The figure shows three views and two pictorial views of one solid part (mm, origin at its lowest corner). Answer the questions. A direction names the side the tool comes from. Give positions to 0.01 mm unless a question says otherwise; leave off trailing zeros. Loops run counter-clockwise (first coordinate to the right, second up) from the corner with the lowest first, then second, coordinate; pieces in that order, holes last. Notation, with made-up numbers: (-6.75, 79.5) - (2.25, 79.5) arc R17 ccw to (2.25, 100.5) - close; hole circle Ø10 at (7, 68). An arc over 180 degrees is marked (long way). One line per question, with ' | ' between items.
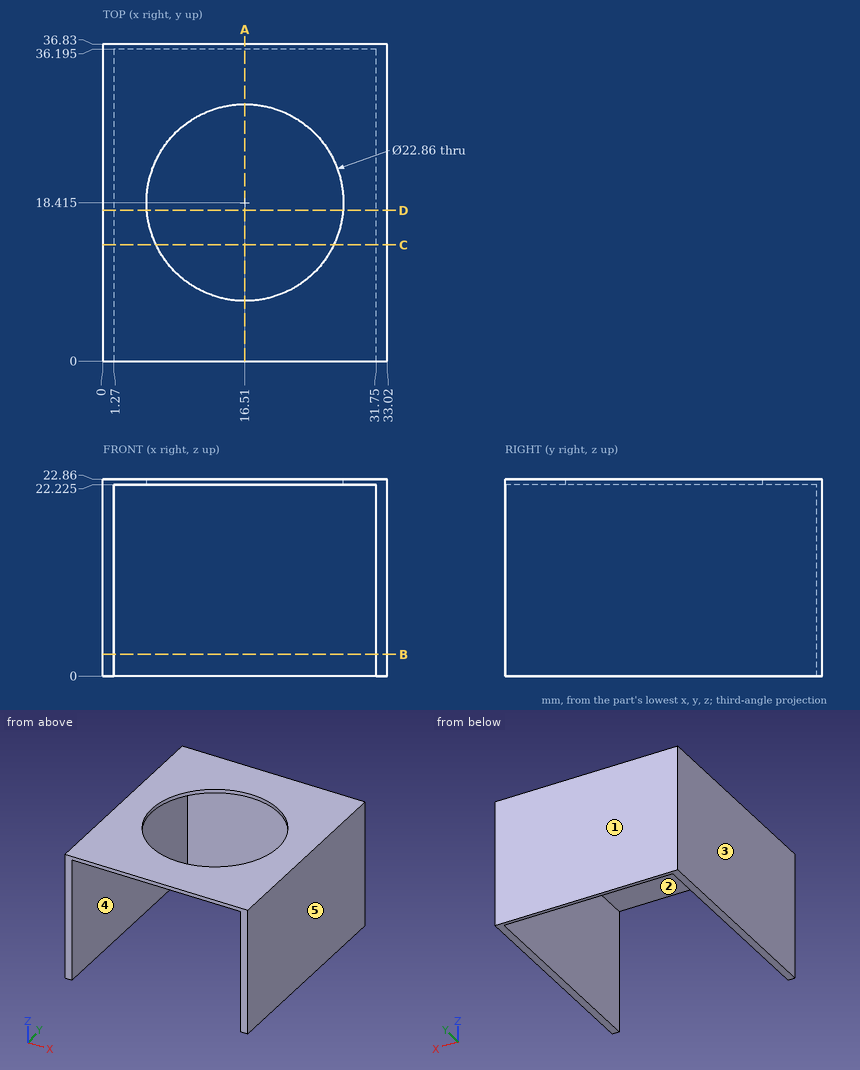
1. Find section C-C on y = 13.5. Write down the section's boundary in (x, z) (3 decimals), then the cut area to 3 significant figures.
Evaluation:
outline: (0, 0) - (1.27, 0) - (1.27, 22.225) - (6.191, 22.225) - (6.191, 22.86) - (0, 22.86) - close; (26.829, 22.225) - (31.75, 22.225) - (31.75, 0) - (33.02, 0) - (33.02, 22.86) - (26.829, 22.86) - close | area: 64.3 mm2
2. Flat-ended cylindrical pins translate along their axes: pin 1 (4 mm diameter, centred on x = 10, z = 12.5, fed in from -Y) (3 decimals); pin 2 (5 mm diameter, centred on x = 8, y = 31.5, fed in from -Z) (3 decimals). Find the tip coordinate at first contact, or state that the pin passes through.
Evaluation:
pin 1: y = 36.195 | pin 2: z = 22.225
3. Consider L1, parallel to X at y = 29.5, z = 2.5; L2, parallel to Y at x = 16.51, z = 22.55 (3 decimals); L3, parallel to Y at x = 31, z = 2.75 (3 decimals). Determine where each line is inside the solid, lowest interval first.
Evaluation:
L1: 0 to 1.27, 31.75 to 33.02 | L2: 0 to 6.985, 29.845 to 36.83 | L3: 36.195 to 36.83
4. Find section B-B on z = 2.5. Write down the section's boundary in (x, y) (3 decimals), then the cut area to 3 significant figures.
Evaluation:
outline: (0, 0) - (1.27, 0) - (1.27, 36.195) - (31.75, 36.195) - (31.75, 0) - (33.02, 0) - (33.02, 36.83) - (0, 36.83) - close | area: 113 mm2
5. Find section D-D on y = 17.5. Write down the section's boundary in (x, z) (3 decimals), then the cut area to 3 significant figures.
Evaluation:
outline: (0, 0) - (1.27, 0) - (1.27, 22.225) - (5.117, 22.225) - (5.117, 22.86) - (0, 22.86) - close; (27.903, 22.225) - (31.75, 22.225) - (31.75, 0) - (33.02, 0) - (33.02, 22.86) - (27.903, 22.86) - close | area: 62.9 mm2
6. Which of the six approach directions +Z, -Z, +X, -X, +Y, -Y give full straight-line access (tool end or side, diameter ignored) to the marked faces 4 and 5?
Evaluation:
face 4: -Z, -Y | face 5: +Z, -Z, +X, +Y, -Y
7. Find section A-A on x = 16.51. Write down the section's boundary in (y, z) (3 decimals).
Evaluation:
outline: (0, 22.225) - (6.985, 22.225) - (6.985, 22.86) - (0, 22.86) - close; (29.845, 22.225) - (36.195, 22.225) - (36.195, 0) - (36.83, 0) - (36.83, 22.86) - (29.845, 22.86) - close
8. Determine the mould class of the marked faces 1, 2 and 3 for opening direction X: +X half, -X half, draft (parallel to the pull), parting line (faces both ways), or undercut.
Evaluation:
face 1: draft | face 2: undercut | face 3: -X half
